from build123d import *

# Parameters (mm, degrees)
SKETCH1_R               = 7.75
BOSS_EXTRUDE1_DEPTH     = 3
BOSS_EXTRUDE2_START     = 4
SKETCH2_R               = 15
BOSS_EXTRUDE2_DEPTH     = 4
CUT_EXTRUDE1_DEPTH      = 104.81508538
CUT_EXTRUDE1_DEPTH_BACK = 104.81508538
SKETCH2_3_R             = 1.7


with BuildPart() as part:
    # Sketch1 → Boss-Extrude1 (new body)
    with BuildSketch(Plane.XY.offset(3)):
        with BuildLine():
            Line((-42.810452402, 40.800302889), (-82.185452402, 35.839519181))
            ThreePointArc((-82.185452402, 35.839519181), (-95.310452402, 20.957168056), (-82.185452402, 6.074816932))
            Line((-82.185452402, 6.074816932), (-42.810452402, 1.114033223))
            ThreePointArc((-42.810452402, 1.114033223), (-20.310452402, 20.957168056), (-42.810452402, 40.800302889))
        make_face()
        with Locations((-40.310452402, 20.957168056)):
            Circle(SKETCH1_R, mode=Mode.SUBTRACT)
    extrude(amount=-BOSS_EXTRUDE1_DEPTH)

    # Sketch2 → Boss-Extrude2 (add)
    with BuildSketch(Plane.XY.offset(3).offset(BOSS_EXTRUDE2_START)):
        with Locations((-80.310452402, 20.957168056)):
            Circle(SKETCH2_R)
    extrude(amount=-BOSS_EXTRUDE2_DEPTH)

    # Sketch2<3> → Cut-Extrude1 (cut, two sides: drawn at the far end of the back side and taken through both)
    with BuildSketch(Plane.XY.offset(3).offset(-CUT_EXTRUDE1_DEPTH_BACK)):
        with Locations((-86.310452402, 20.957168056)):
            Circle(SKETCH2_3_R)
        with Locations((-80.310452402, 26.957168056)):
            Circle(SKETCH2_3_R)
        with Locations((-74.310452402, 20.957168056)):
            Circle(SKETCH2_3_R)
        with Locations((-80.310452402, 14.957168056)):
            Circle(SKETCH2_3_R)
    extrude(amount=CUT_EXTRUDE1_DEPTH + CUT_EXTRUDE1_DEPTH_BACK, mode=Mode.SUBTRACT)


solid = part.part
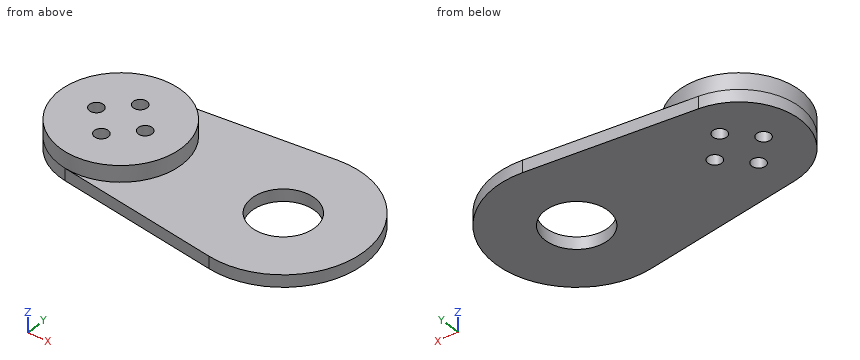
Input: part model. Units: mm. Frame: model coordinates. Give positions to 0.01 mm unless a question says otherwise; leave off trailing zeros. Order: outer loops, then holes, each group sorted by start corner. A loop starts at its lowest first (then second) coordinate and runs counter-clockwise, first axis right, second up. Notation, with made-up numbers: (4, -39) - (53, -39) arc R17 ccw to (53, -14) - close; hole circle Ø5 at (16.5, 27.5). An arc over 180 degrees is marked (long way). Write each question's results on one line, items separated by ' | '.
Item 1: Section B-B (z = 2.25). Return loops of the section in (x, y), and give its area (3 significant figures).
A:
outline: (-82.19, 6.07) - (-42.81, 1.11) arc R20 ccw (long way) to (-42.81, 40.8) - (-82.19, 35.84) arc R15 ccw to start; hole circle Ø3.4 at (-86.31, 20.96); hole circle Ø3.4 at (-80.31, 14.96); hole circle Ø3.4 at (-80.31, 26.96); hole circle Ø3.4 at (-74.31, 20.96); hole circle Ø15.5 at (-40.31, 20.96) | area: 2,170 mm^2
Item 2: Section D-D (x = -45.5). Return loops of the section in (y, z).
A:
outline: (1.45, 0) - (15.2, 0) - (15.2, 3) - (1.45, 3) - close; (26.71, 0) - (40.46, 0) - (40.46, 3) - (26.71, 3) - close
Item 3: Section A-A (x = -73.5). Return loops of the section in (y, z).
A:
outline: (4.98, 0) - (19.46, 0) - (19.46, 7) - (7.59, 7) - (7.59, 3) - (4.98, 3) - close; (22.45, 0) - (36.93, 0) - (36.93, 3) - (34.32, 3) - (34.32, 7) - (22.45, 7) - close
Item 4: Section C-C (y = 11). Return loops of the section in (x, z), and give its area (3 significant figures).
A:
outline: (-91.53, 0) - (-22.97, 0) - (-22.97, 3) - (-69.09, 3) - (-69.09, 7) - (-91.53, 7) - close | area: 295 mm^2
Item 5: Material intervals for line 1 along X through (y, z) = (16, 2.5); line 2 along Y through (x, z) = (-80, 2.25); line 3 along Y through (x, z) = (-74, 4.25), sorted ascending.
A:
line 1: x = -94.47 to -81.65, -78.97 to -46.27, -34.35 to -20.93 | line 2: y = 5.8 to 13.29, 16.63 to 25.29, 28.63 to 36.11 | line 3: y = 7.35 to 19.29, 22.63 to 34.57
Item 6: Contact query for flat-ended pins moving along their axis: pin 1 Ø10 at (x, y) = (-50, 14) entering from +Z; pin 2 Ø2 at (x, y) = (-80.31, 14.96) entering from -Z. Output: stop coordinate, or through.
A:
pin 1: stops at z = 3 | pin 2: passes through
